```python
from build123d import *

# Parameters (mm, degrees)
F1_DEPTH = 200


with BuildPart() as f1:
    # F0 (on Front) → F1 (new body)
    with BuildSketch(Plane.XZ):
        with BuildLine():
            Line((12.5, 15), (5.1, 15))
            Line((5.1, 15), (5.1, 13.8))
            Line((5.1, 13.8), (4.1, 13.8))
            Line((4.1, 13.8), (4.1, 12.6))
            Line((4.1, 12.6), (8.25, 12.6))
            Line((8.25, 12.6), (8.25, 9.664214))
            Line((8.25, 9.664214), (5.092893, 6.507107))
            Line((5.092893, 6.507107), (4.385786, 5.8))
            Line((4.385786, 5.8), (0, 5.8))
            Line((0, 5.8), (-4.385786, 5.8))
            Line((-4.385786, 5.8), (-5.092893, 6.507107))
            Line((-5.092893, 6.507107), (-8.25, 9.664214))
            Line((-8.25, 9.664214), (-8.25, 12.6))
            Line((-8.25, 12.6), (-4.1, 12.6))
            Line((-4.1, 12.6), (-4.1, 13.8))
            Line((-4.1, 13.8), (-5.1, 13.8))
            Line((-5.1, 13.8), (-5.1, 15))
            Line((-5.1, 15), (-12.5, 15))
            ThreePointArc((-12.5, 15), (-14.267767, 14.267767), (-15, 12.5))
            Line((-15, 12.5), (-15, 5.1))
            Line((-15, 5.1), (-13.8, 5.1))
            Line((-13.8, 5.1), (-13.8, 4.1))
            Line((-13.8, 4.1), (-12.6, 4.1))
            Line((-12.6, 4.1), (-12.6, 8.25))
            Line((-12.6, 8.25), (-9.664214, 8.25))
            Line((-9.664214, 8.25), (-6.507107, 5.092893))
            Line((-6.507107, 5.092893), (-5.8, 4.385786))
            Line((-5.8, 4.385786), (-5.8, 0))
            Line((-5.8, 0), (-5.8, -4.385786))
            Line((-5.8, -4.385786), (-6.507107, -5.092893))
            Line((-6.507107, -5.092893), (-9.664214, -8.25))
            Line((-9.664214, -8.25), (-12.6, -8.25))
            Line((-12.6, -8.25), (-12.6, -4.1))
            Line((-12.6, -4.1), (-13.8, -4.1))
            Line((-13.8, -4.1), (-13.8, -5.1))
            Line((-13.8, -5.1), (-15, -5.1))
            Line((-15, -5.1), (-15, -12.5))
            ThreePointArc((-15, -12.5), (-14.267767, -14.267767), (-12.5, -15))
            Line((-12.5, -15), (-5.1, -15))
            Line((-5.1, -15), (-5.1, -13.8))
            Line((-5.1, -13.8), (-4.1, -13.8))
            Line((-4.1, -13.8), (-4.1, -12.6))
            Line((-4.1, -12.6), (-8.25, -12.6))
            Line((-8.25, -12.6), (-8.25, -9.664214))
            Line((-8.25, -9.664214), (-5.092893, -6.507107))
            Line((-5.092893, -6.507107), (-4.385786, -5.8))
            Line((-4.385786, -5.8), (0, -5.8))
            Line((0, -5.8), (4.385786, -5.8))
            Line((4.385786, -5.8), (5.092893, -6.507107))
            Line((5.092893, -6.507107), (8.25, -9.664214))
            Line((8.25, -9.664214), (8.25, -12.6))
            Line((8.25, -12.6), (4.1, -12.6))
            Line((4.1, -12.6), (4.1, -13.8))
            Line((4.1, -13.8), (5.1, -13.8))
            Line((5.1, -13.8), (5.1, -15))
            Line((5.1, -15), (12.5, -15))
            ThreePointArc((12.5, -15), (14.267767, -14.267767), (15, -12.5))
            Line((15, -12.5), (15, -5.1))
            Line((15, -5.1), (13.8, -5.1))
            Line((13.8, -5.1), (13.8, -4.1))
            Line((13.8, -4.1), (12.6, -4.1))
            Line((12.6, -4.1), (12.6, -8.25))
            Line((12.6, -8.25), (9.664214, -8.25))
            Line((9.664214, -8.25), (6.507107, -5.092893))
            Line((6.507107, -5.092893), (5.8, -4.385786))
            Line((5.8, -4.385786), (5.8, 0))
            Line((5.8, 0), (5.8, 4.385786))
            Line((5.8, 4.385786), (6.507107, 5.092893))
            Line((6.507107, 5.092893), (9.664214, 8.25))
            Line((9.664214, 8.25), (12.6, 8.25))
            Line((12.6, 8.25), (12.6, 4.1))
            Line((12.6, 4.1), (13.8, 4.1))
            Line((13.8, 4.1), (13.8, 5.1))
            Line((13.8, 5.1), (15, 5.1))
            Line((15, 5.1), (15, 12.5))
            ThreePointArc((15, 12.5), (14.267767, 14.267767), (12.5, 15))
        make_face()
        with BuildLine():
            ThreePointArc((-3.4, 0), (-2.404163, 2.404163), (0, 3.4))
            ThreePointArc((0, 3.4), (2.404163, 2.404163), (3.4, 0))
            ThreePointArc((3.4, 0), (2.404163, -2.404163), (0, -3.4))
            ThreePointArc((0, -3.4), (-2.404163, -2.404163), (-3.4, 0))
        make_face(mode=Mode.SUBTRACT)
    extrude(amount=F1_DEPTH)


solid = f1.part
```
The listing builds one solid part. Answer for the finished solid, in the listing's coordinates (mm). A direction names the side the tool comes from. Round coordinates to 2 decimals unless told otherwise and drop trailing zeros. Use one line per item in the form item = value. Start each with the question number.
1. Consider line 1 (Z direction, x = -8, y = -143); line 2 (X direction, y = -34, z = -4.5); line 3 (X direction, y = -35.5, z = -5.5). Determine where each line is inside the solid, lowest interval first. Write a range as [from, to].
2. For a pull along Z with two mould halves and no side action, classify faces 1 (the face through (-15, -99, -9)), 2 (the face through (9, -99, 15)), 3 (the face through (-6, -99, 12.6)) as pulls with the +Z half, pulls with the -Z half, needs draft (parallel to the pull), parting line crosses it, or undercut.
3. A tool of negligible diameter and unlimited length cuts with its end or side. For faces 4 (the face through (0, 0, 4)), 5 (the face through (-12.6, -99, -6)), from which of +Z, -Z, +X, -X, +Y, -Y can it reach the whole face along a straight path? Write none if from no direction.
4. Given pin 1 Ø0.5 at (x, y) = (4.5, -115) entering from +Z; pin 2 Ø1.5 at (y, z) = (-49, -1) entering from -X; pin 3 Ø5 at (x, z) = (-10.5, 7) entering from -Y; pin 4 Ø1.3 at (y, z) = (-122.5, -14.5) entering from +X, each flat-ended and moving along its own axis, determine where each tip first touches the part or whether it passes through.
Geometry check:
q1.line_1 = [-15, -12.6], [-9.41, -6.59], [6.59, 9.41], [12.6, 15]
q1.line_2 = [-13.8, -12.6], [-5.91, 5.91], [12.6, 13.8]
q1.line_3 = [-15, -12.6], [-6.91, 6.91], [12.6, 15]
q2.face_1 = needs draft
q2.face_2 = pulls with the +Z half
q2.face_3 = undercut
q3.face_4 = +Z, -Z, +X, -X, +Y
q3.face_5 = +Y, -Y
q4.pin_1 = 13.8
q4.pin_2 = -5.8
q4.pin_3 = -200
q4.pin_4 = 14.6
